CAD build for the part. Positions are in the model's coordinates, mm. Face numbers are marked on the shaded views. A direction names the side the tool comes from. Give positions to 0.01 mm unless a question says otherwise; leave off trailing zeros. Order: outer loops, then holes, each group sorted by start corner. A loop starts at its lowest first (then second) coordinate and runs counter-clockwise, first axis right, second up.
```python
from build123d import *

# Parameters (mm, degrees)
SKETCH006_W  = 14
SKETCH006_H  = 0.6
PAD018_DEPTH = 9.6
PAD019_DEPTH = 9
PAD020_DEPTH = 6.4
PAD021_DEPTH = 4.4
SKETCH010_W  = 0.6
SKETCH010_H  = 0.6
PAD022_DEPTH = 3.5


with BuildPart() as part:
    # Sketch006 → Pad018 (new body)
    with BuildSketch(Plane.YZ.offset(16)):
        with Locations((0, 3.5)):
            Rectangle(SKETCH006_W, SKETCH006_H)
    extrude(amount=PAD018_DEPTH)

    # Sketch036 → Pad019 (join)
    with BuildSketch(Plane.YZ.offset(16)):
        Polygon((7.8, 8.8), (7.8, 3.8), (0.5, 3.8), (0, 3.4), (-0.5, 3.8), (-7.8, 3.8), (-7.8, 8.8), (-7.3, 8.8), (-7.3, 4.2), (7.3, 4.2), (7.3, 8.8), align=None)
    extrude(amount=PAD019_DEPTH)

    # Sketch037 → Pad020 (join)
    with BuildSketch(Plane.YZ.offset(16)):
        Polygon((-7, 9.4), (7, 9.4), (7, 4.2), (6.1, 4.2), (6.1, 4.5), (-6.1, 4.5), (-6.1, 4.2), (-7, 4.2), align=None)
    extrude(amount=PAD020_DEPTH)

    # Sketch038 (on Face21 of Pad020) → Pad021 (join)
    with BuildSketch(Plane.YZ.offset(22.4)):
        Polygon((-7, 9.4), (-4, 9.4), (-4, 8.8), (-6.4, 8.8), (-6.4, 7.8), (-7, 7.8), align=None)
        Polygon((4, 9.4), (7, 9.4), (7, 7.8), (6.4, 7.8), (6.4, 8.8), (4, 8.8), align=None)
        Polygon((7, 7), (7, 4.2), (6.1, 4.2), (6.1, 4.5), (-6.1, 4.5), (-6.1, 4.2), (-7, 4.2), (-7, 7), (-6.4, 7), (-6.4, 5.3), (6.4, 5.3), (6.4, 7), align=None)
    extrude(amount=PAD021_DEPTH)

    # Sketch010 (on Face35 of Pad021) → Pad022 (join)
    with BuildSketch(Plane.YZ.offset(22.4)):
        with Locations((-5, 7.4)):
            Rectangle(SKETCH010_W, SKETCH010_H)
        with Locations((-3, 7.4)):
            Rectangle(SKETCH010_W, SKETCH010_H)
        with Locations((-1, 7.4)):
            Rectangle(SKETCH010_W, SKETCH010_H)
        with Locations((1, 7.4)):
            Rectangle(SKETCH010_W, SKETCH010_H)
        with Locations((3, 7.4)):
            Rectangle(SKETCH010_W, SKETCH010_H)
        with Locations((5, 7.4)):
            Rectangle(SKETCH010_W, SKETCH010_H)
    extrude(amount=PAD022_DEPTH)


solid = part.part
```
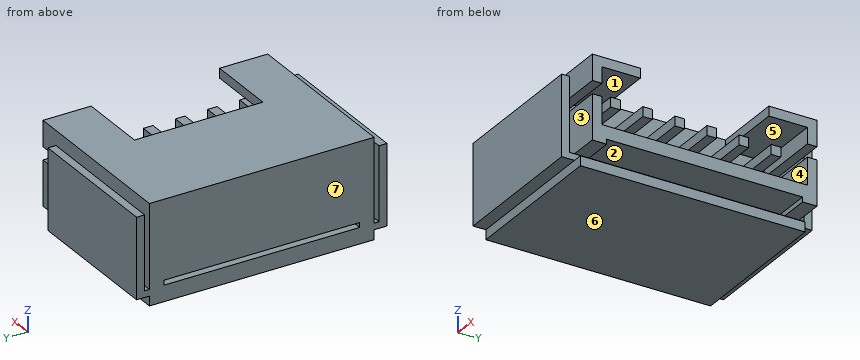
Item 1: Two-plate mould, pull along Z, no slides. Class the marked faces 4, 5, 6 and 7: released by +Z, released by -Z, zero draft, split by the parting line, or undercut.
Item 2: Slice it at D-D (x = 20). Give the cut face in (y, z).
Item 3: Slice it at C-C (y = 4.5). Give the cut face in (x, z), and give its area (3 significant figures).
Item 4: Tool access for the marked faces 1, 2 and 3: list every direction of +Z, -Z, +X, -X, +Y, -Y with a clear straight run to the whole face (end or side of a thin tool).
Item 5: Slice it at B-B (x = 26.25). Give the cut face in (y, z).
Item 6: Drop flat-ended pins along their axis: pin 1 Ø0.5 at (y, z) = (1, 7.5) entering from +X; pin 2 Ø0.7 at (x, y) = (26, -7) entering from -Z. Give the stop position or say it passes through.
Item 7: Wall check: L1, parallel to Y at x = 18.5, z = 4.25; L2, parallel to Y at x = 17.5, z = 7.5; L3, parallel to Z at x = 24.25, y = 4.75. Give the ranges that are in metal, low to high.
Item 8: Slice it at A-A (z = 5). Give the cut face in (x, y), and give its area (3 significant figures).
A:
1. face 4: undercut
1. face 5: undercut
1. face 6: released by -Z
1. face 7: zero draft
2. outline: (-7.8, 3.8) - (-7, 3.8) - (-7, 3.2) - (7, 3.2) - (7, 3.8) - (7.8, 3.8) - (7.8, 8.8) - (7.3, 8.8) - (7.3, 4.2) - (7, 4.2) - (7, 9.4) - (-7, 9.4) - (-7, 4.2) - (-7.3, 4.2) - (-7.3, 8.8) - (-7.8, 8.8) - close; hole (-6.1, 4.2) - (6.1, 4.2) - (6.1, 4.5) - (-6.1, 4.5) - close
3. outline: (16, 3.2) - (25.6, 3.2) - (25.6, 3.8) - (25, 3.8) - (25, 4.2) - (16, 4.2) - close; (16, 4.5) - (26.8, 4.5) - (26.8, 5.3) - (22.4, 5.3) - (22.4, 8.8) - (26.8, 8.8) - (26.8, 9.4) - (16, 9.4) - close
3. area: 46.9 mm2
4. face 1: +X
4. face 2: +X, -X
4. face 3: +Z, +X, -X
5. outline: (-7, 4.2) - (-6.1, 4.2) - (-6.1, 4.5) - (6.1, 4.5) - (6.1, 4.2) - (7, 4.2) - (7, 7) - (6.4, 7) - (6.4, 5.3) - (-6.4, 5.3) - (-6.4, 7) - (-7, 7) - close; (-7, 7.8) - (-6.4, 7.8) - (-6.4, 8.8) - (-4, 8.8) - (-4, 9.4) - (-7, 9.4) - close; (4, 8.8) - (6.4, 8.8) - (6.4, 7.8) - (7, 7.8) - (7, 9.4) - (4, 9.4) - close
6. pin 1: stops at x = 25.9
6. pin 2: stops at z = 4.2
7. L1: y = -7.8 to -7.3, -7 to -6.1, 6.1 to 7, 7.3 to 7.8
7. L2: y = -7.8 to -7.3, -7 to 7, 7.3 to 7.8
7. L3: z = 3.2 to 4.2, 4.5 to 5.3, 7.1 to 7.7, 8.8 to 9.4
8. outline: (16, -7.8) - (25, -7.8) - (25, -7.3) - (16, -7.3) - close; (16, -7) - (26.8, -7) - (26.8, 7) - (16, 7) - close; (16, 7.3) - (25, 7.3) - (25, 7.8) - (16, 7.8) - close
8. area: 160 mm2
